from build123d import *

# Parameters (mm, degrees)
SKETCH_1_R       = 1.15
SKETCH_1_R_2     = 0.939967297
SKETCH_1_R_3     = 0.967686678
SKETCH_1_R_4     = 1.65
SKETCH_1_W       = 30.4982
SKETCH_1_H       = 42.7098
SKETCH_1_W_2     = 3
SKETCH_1_H_2     = 24
PIXHAWK_M3_DEPTH = 1.5


with BuildPart() as part:
    # 草图1 → Pixhawk正装减振托板_绑带槽_四M3孔 (new body)
    with BuildSketch(Plane.XY):
        Polygon((24, -39), (24, -43), (18, -49), (-18, -49), (-24, -43), (-24, -39), (-30, -33), (-30, 33), (-24, 39), (-24, 43), (-18, 49), (18, 49), (24, 43), (24, 39), (30, 33), (30, -33), align=None)
        with Locations((16, 30)):
            Circle(SKETCH_1_R, mode=Mode.SUBTRACT)
        with Locations((-16, -30)):
            Circle(SKETCH_1_R, mode=Mode.SUBTRACT)
        with Locations((16, -30)):
            Circle(SKETCH_1_R_2, mode=Mode.SUBTRACT)
        with Locations((-16, 30)):
            Circle(SKETCH_1_R_3, mode=Mode.SUBTRACT)
        with Locations((-27, -30)):
            Circle(SKETCH_1_R_4, mode=Mode.SUBTRACT)
        with Locations((-27, 30)):
            Circle(SKETCH_1_R_4, mode=Mode.SUBTRACT)
        with Locations((27, -30)):
            Circle(SKETCH_1_R_4, mode=Mode.SUBTRACT)
        with Locations((27, 30)):
            Circle(SKETCH_1_R_4, mode=Mode.SUBTRACT)
        Rectangle(SKETCH_1_W, SKETCH_1_H, mode=Mode.SUBTRACT)
        with Locations((-26, 0)):
            Rectangle(SKETCH_1_W_2, SKETCH_1_H_2, mode=Mode.SUBTRACT)
        with Locations((26, 0)):
            Rectangle(SKETCH_1_W_2, SKETCH_1_H_2, mode=Mode.SUBTRACT)
    extrude(amount=PIXHAWK_M3_DEPTH)


solid = part.part
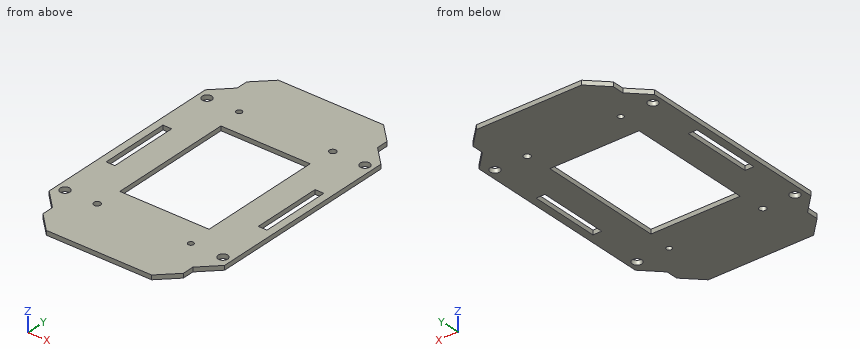
Model file for the job. Use its own axes, mm. Coordinates: 2 decimals unless noted, no trailing zeros. Order: outer loops, then holes, each group sorted by start corner. A loop starts at its lowest first (then second) coordinate and runs counter-clockwise, first axis right, second up. Notation, with made-up numbers: (-23.5, 65.5) -> (-9.5, 65.5) arc R10 ccw to (-9.5, 71.5) -> close; hole circle Ø10 at (68, 47.5). An arc over 180 degrees is marked (long way). Return JSON: item names as keys, results as strings. Group by question number.
Item 1: Saw through at D-D on y = 15. Write the cut outline in (x, z).
Item 2: Saw through at B-B on y = 30. Write the cut outline in (x, z), then the cut area to 3 significant figures.
Item 3: Saw through at C-C on x = -7. Write the cut outline in (y, z).
Item 4: Flat gauge pins, fed straight in: P1, Ø1.1, axis at x = 16, y = -30, coming from the -Z side; P2, Ø5.5, axis at x = 27, y = -30, coming from the -Z side; P3, Ø0.8, axis at y = -41.5, z = 1, coming from the -X side. Where does each tip first touch, or does it go through?
Item 5: Saw through at A-A on y = 3.5. Write the cut outline in (x, z), then the cut area to 3 significant figures.
Item 6: Wall check: line 1 along X through (y, z) = (5, 0.15); line 2 along Y through (x, z) = (10, 0.35); line 3 along Y through (x, z) = (27, 0.5). Give the ranges that are in metal, low to high. Write a range as [from, to].
Values found:
{
 "1": {"outline": "(-30, 0) -> (-15.25, 0) -> (-15.25, 1.5) -> (-30, 1.5) -> close; (15.25, 0) -> (30, 0) -> (30, 1.5) -> (15.25, 1.5) -> close"},
 "2": {"outline": "(-30, 0) -> (-28.65, 0) -> (-28.65, 1.5) -> (-30, 1.5) -> close; (-25.35, 0) -> (-16.97, 0) -> (-16.97, 1.5) -> (-25.35, 1.5) -> close; (-15.03, 0) -> (14.85, 0) -> (14.85, 1.5) -> (-15.03, 1.5) -> close; (17.15, 0) -> (25.35, 0) -> (25.35, 1.5) -> (17.15, 1.5) -> close; (28.65, 0) -> (30, 0) -> (30, 1.5) -> (28.65, 1.5) -> close", "area": "73.7 mm2"},
 "3": {"outline": "(-49, 0) -> (-21.35, 0) -> (-21.35, 1.5) -> (-49, 1.5) -> close; (21.35, 0) -> (49, 0) -> (49, 1.5) -> (21.35, 1.5) -> close"},
 "4": {"P1": "passes through", "P2": "stops at z = 0", "P3": "stops at x = -24"},
 "5": {"outline": "(-30, 0) -> (-27.5, 0) -> (-27.5, 1.5) -> (-30, 1.5) -> close; (-24.5, 0) -> (-15.25, 0) -> (-15.25, 1.5) -> (-24.5, 1.5) -> close; (15.25, 0) -> (24.5, 0) -> (24.5, 1.5) -> (15.25, 1.5) -> close; (27.5, 0) -> (30, 0) -> (30, 1.5) -> (27.5, 1.5) -> close", "area": "35.3 mm2"},
 "6": {"line 1": "x = [-30, -27.5], [-24.5, -15.25], [15.25, 24.5], [27.5, 30]", "line 2": "y = [-49, -21.35], [21.35, 49]", "line 3": "y = [-36, -31.65], [-28.35, -12], [12, 28.35], [31.65, 36]"}
}
